Part model, mm, in its own coordinate system. A direction names the side the tool comes from. Round coordinates to 2 decimals unless told otherwise and drop trailing zeros. Order: outer loops, then holes, each group sorted by start corner. A loop starts at its lowest first (then second) coordinate and runs counter-clockwise, first axis right, second up. Notation, with made-up numbers: (67, 46.5) -> (93, 46.5) arc R32 ccw to (93, 84.5) -> close; hole circle Ø3 at (17, 58.5). An arc over 180 degrees is marked (long way). Return JSON: item names as keys, results as strings. Group by question number.
from build123d import *

# Parameters (mm, degrees)
F1_DEPTH = 3
F2_DEPTH = 25
F3_R     = 3


with BuildPart() as f1:
    # F0 (on Top) → F1 (new body)
    with BuildSketch(Plane.XY):
        Polygon((34.9999997169, -20.9999997169), (34.9999997169, 4.9999997169), (4.9999997169, 4.9999997169), (4.9999997169, 63.9999997169), (-20.9999997169, 63.9999997169), (-20.9999997169, -20.9999997169), align=None)
        Polygon((0, 59), (0, 0), (30, 0), (30, -16), (-16, -16), (-16, 59), align=None, mode=Mode.SUBTRACT)
        Polygon((30, 0), (0, 0), (0, 59), (-16, 59), (-16, -16), (30, -16), align=None)
        Polygon((-15.3, 58.3), (-0.7, 58.3), (-0.7, -0.7), (29.3, -0.7), (29.3, -15.3), (-15.3, -15.3), align=None, mode=Mode.SUBTRACT)
        Polygon((-0.7, -0.7), (-0.7, 58.3), (-15.3, 58.3), (-15.3, -15.3), (29.3, -15.3), (29.3, -0.7), align=None)
        Polygon((28.3, -1.7), (28.3, -14.3), (-14.3, -14.3), (-14.3, 57.3), (-1.7, 57.3), (-1.7, -1.7), align=None, mode=Mode.SUBTRACT)
    extrude(amount=F1_DEPTH)

    # F0 (on Top) → F2 (join)
    with BuildSketch(Plane.XY):
        Polygon((30, 0), (0, 0), (0, 59), (-16, 59), (-16, -16), (30, -16), align=None)
        Polygon((-15.3, 58.3), (-0.7, 58.3), (-0.7, -0.7), (29.3, -0.7), (29.3, -15.3), (-15.3, -15.3), align=None, mode=Mode.SUBTRACT)
    extrude(amount=F2_DEPTH)

    # F3
    f3_edges = [f1.edges().sort_by_distance(p)[0] for p in [
        (35, -21, 1.5),
        (35, 5, 1.5),
        (5, 5, 1.5),
        (5, 64, 1.5),
        (-21, 64, 1.5),
        (-21, -21, 1.5),
        (-14.3, -14.3, 1.5),
        (-1.7, -1.7, 1.5),
        (28.3, -14.3, 1.5),
        (28.3, -1.7, 1.5),
        (-1.7, 57.3, 1.5),
        (-14.3, 57.3, 1.5),
    ]]
    fillet(f3_edges, radius=F3_R)


solid = f1.part
(1) Probe L1, parallel to Y at x = -8, z = 14; L2, parallel to X at y = 25, z = 6.25. List the from-to ranges inside material, lowest first. Write a range as [from, to].
(2) Saw through at C-C, the plane z = 12.25. List the corners of the cut face in (x, y), and give its area (3 significant figures).
(3) Tool access for faces 1 (the flat face through (-16, 22, 14)), 2 (the cylindrical face through (-13.4, 56.44, 1.52)), 3 (the flat face through (7, -15.3, 14)), 4 (the flat face through (15, 0, 14)), 5 (the flat face through (5, 34, 1)): list every direction of +Z, -Z, +X, -X, +Y, -Y with a clear straight run to the whole face (end or side of a thin tool).
(4) Pin check, flat tips, straight feed: P1, Ø10, axis at y = 16, z = 12.5, coming from the -X side; P2, Ø11, axis at x = 22, z = 13.5, coming from the +Y side; P3, Ø11, axis at y = 20.5, z = 19.5, coming from the +X side. Stop position of each tip, or through.
(5) Saw through at A-A, the plane x = 11. List the corners of the cut face in (y, z), and give its area (3 significant figures).
Results are:
{
 "1": {"L1": "y = [-16, -15.3], [58.3, 59]", "L2": "x = [-16, -15.3], [-0.7, 0]"},
 "2": {"outline": "(-16, -16) -> (30, -16) -> (30, 0) -> (0, 0) -> (0, 59) -> (-16, 59) -> close; hole (-15.3, -15.3) -> (29.3, -15.3) -> (29.3, -0.7) -> (-0.7, -0.7) -> (-0.7, 58.3) -> (-15.3, 58.3) -> close", "area": "167 mm^2"},
 "3": {"face 1": "+Z, -X, +Y, -Y", "face 2": "+Z, -Z", "face 3": "+Z", "face 4": "+Z, +X, +Y", "face 5": "+Z, -Z, +X, +Y"},
 "4": {"P1": "stops at x = -16", "P2": "stops at y = 0", "P3": "stops at x = 0"},
 "5": {"outline": "(-21, 0) -> (-14.3, 0) -> (-14.3, 3) -> (-15.3, 3) -> (-15.3, 25) -> (-16, 25) -> (-16, 3) -> (-21, 3) -> close; (-1.7, 0) -> (5, 0) -> (5, 3) -> (0, 3) -> (0, 25) -> (-0.7, 25) -> (-0.7, 3) -> (-1.7, 3) -> close", "area": "71.0 mm^2"}
}
